Read the model definition and answer for the solid it produces. Units are mm, in the model's axes. Give positions to 0.01 mm unless a question says otherwise; leave off trailing zeros. Put each result on its own line as item: value. Start each with the question number.
1. A cutting plane is placed at B-B, the plane y = 0. Count the separate pieces of the cut face and the enclosed holes in it, plus the area to 3 significant figures.
2. Given pin 1 Ø6.5 at (x, y) = (-16.5, 2) entering from +Z; pin 2 Ø4 at (x, y) = (-20, -3.5) entering from -Z, each flat-ended and moving along its own axis, determine where each tip first touches the part or whether it passes through.
3. Consider L1, parallel to X at y = 0, z = 1.25; L2, parallel to X at y = 4, z = 0.6; L3, parallel to Y at x = 19.05, z = 1.25. Determine where each line is inside the solid, lowest interval first. Write a range as from..to.
```python
from build123d import *

# Parameters (mm, degrees)
SKETCH_W     = 76.2
SKETCH_H     = 25.4
SKETCH_R     = 4.7625
PAD_DEPTH    = 1.905
SKETCH001_W  = 12.7
SKETCH001_H  = 12.7
POCKET_DEPTH = 0.254
CHAMFER_SIZE = 1
FILLET_R     = 1


with BuildPart() as part:
    # Sketch → Pad (new body)
    with BuildSketch(Plane.XY):
        Rectangle(SKETCH_W, SKETCH_H)
        with Locations((-19.05, 0)):
            Circle(SKETCH_R, mode=Mode.SUBTRACT)
        with Locations((19.05, 0)):
            Circle(SKETCH_R, mode=Mode.SUBTRACT)
    extrude(amount=PAD_DEPTH)

    # Sketch001 → Pocket (cut)
    with BuildSketch(Plane.XY.offset(1.905)):
        with Locations((-19.05, 0)):
            Rectangle(SKETCH001_W, SKETCH001_H)
        with Locations((19.05, 0)):
            Rectangle(SKETCH001_W, SKETCH001_H)
    extrude(amount=-POCKET_DEPTH, mode=Mode.SUBTRACT)

    # Chamfer
    chamfer_edges = [part.edges().sort_by_distance(p)[0] for p in [
        (14.2875, 0, 0),
        (-23.8125, 0, 0),
    ]]
    chamfer(chamfer_edges, length=CHAMFER_SIZE)

    # Fillet
    fillet_edges = [part.edges().sort_by_distance(p)[0] for p in [
        (38.1, 12.7, 0.9525),
        (38.1, -12.7, 0.9525),
        (-38.1, -12.7, 0.9525),
        (-38.1, 12.7, 0.9525),
    ]]
    fillet(fillet_edges, radius=FILLET_R)


solid = part.part
```
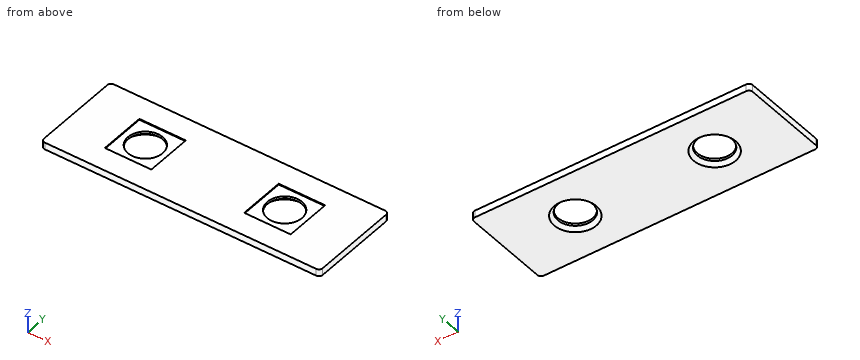
Return value:
1. separate pieces: 3
1. enclosed holes: 0
1. area: 105 mm2
2. pin 1: stops at z = 1.65
2. pin 2: stops at z = 0.14
3. L1: x = -38.1..-23.81, -14.29..14.29, 23.81..38.1
3. L2: x = -38.1..-22.31, -15.79..15.79, 22.31..38.1
3. L3: y = -12.7..-4.76, 4.76..12.7
